Model file for the job. Use its own axes, mm. Coordinates: 2 decimals unless noted, no trailing zeros. Order: outer loops, then holes, each group sorted by start corner. A loop starts at its lowest first (then second) coordinate and runs counter-clockwise, first axis right, second up. Notation, with made-up numbers: M 62,20.25 L 112,20.25 A29 cw 112,49.25 Z; hole C 86,-26.75 d3. An arc over 180 degrees is marked long. Return JSON: item names as keys, results as strings.
```python
from build123d import *

# Parameters (mm, degrees)
SKETCH2_W           = 17
SKETCH2_H           = 5
BOSS_EXTRUDE1_DEPTH = 5
SKETCH3_R           = 1.5
SKETCH3_R_2         = 1.45
SKETCH3_R_3         = 1.55
SKETCH3_R_4         = 1.525
SKETCH3_R_5         = 1.475
CUT_EXTRUDE1_DEPTH  = 6
SKETCH4_W           = 5
SKETCH4_H           = 5
BOSS_EXTRUDE2_DEPTH = 1.5
SKETCH5_W           = 5
SKETCH5_H           = 5
BOSS_EXTRUDE3_DEPTH = 1.5
FILLET1_R           = 0.5


with BuildPart() as part:
    # Sketch2 → Boss-Extrude1 (new body)
    with BuildSketch(Plane(origin=(0, 0, 0), x_dir=(1, 0, 0), z_dir=(0, 1, 0))):
        with Locations((1.12006706, -0.094563726)):
            Rectangle(SKETCH2_W, SKETCH2_H)
    extrude(amount=BOSS_EXTRUDE1_DEPTH)

    # Sketch3 → Cut-Extrude1 (cut, through all)
    with BuildSketch(Plane(origin=(0, 5, 0), x_dir=(1, 0, 0), z_dir=(0, 1, 0))):
        with Locations((1.12006706, -0.094563726)):
            Circle(SKETCH3_R)
        with Locations((7.97006706, -0.094563726)):
            Circle(SKETCH3_R_2)
        with Locations((-5.72993294, -0.094563726)):
            Circle(SKETCH3_R_3)
        with Locations((-2.354549871, -0.094563726)):
            Circle(SKETCH3_R_4)
        with Locations((4.597069825, -0.094563726)):
            Circle(SKETCH3_R_5)
    extrude(amount=-CUT_EXTRUDE1_DEPTH, mode=Mode.SUBTRACT)

    # Sketch4 → Boss-Extrude2 (add)
    with BuildSketch(Plane.ZY.offset(7.37993294)):
        with Locations((0.094563726, 2.5)):
            Rectangle(SKETCH4_W, SKETCH4_H)
    extrude(amount=BOSS_EXTRUDE2_DEPTH)

    # Sketch5 → Boss-Extrude3 (add)
    with BuildSketch(Plane(origin=(9.62006706, 0, 0), x_dir=(0, 0, -1), z_dir=(1, 0, 0))):
        with Locations((-0.094563726, 2.5)):
            Rectangle(SKETCH5_W, SKETCH5_H)
    extrude(amount=BOSS_EXTRUDE3_DEPTH)

    # Fillet1
    fillet1_edges = [part.edges().sort_by_distance(p)[0] for p in [
        (1.12006706, 5, -2.405436274),
        (-8.87993294, 2.5, -2.405436274),
        (-8.87993294, 2.5, 2.594563726),
        (-8.87993294, 5, 0.094563726),
        (11.12006706, 2.5, 2.594563726),
        (11.12006706, 2.5, -2.405436274),
        (11.12006706, 5, 0.094563726),
        (1.12006706, 5, 2.594563726),
    ]]
    fillet(fillet1_edges, radius=FILLET1_R)


solid = part.part
```
Item 1: Pull direction Z, two halves, no side cores. Call faces 1 (the flat face through (1, 2, -2.405)), 2 (the cylindrical face through (-4.25, 2.54, -0.37)), 3 (the flat face through (1, 2, 2.595)), 4 (the flat face through (1, 0, -2)): +Z half, -Z half, draft (parallel to the pull), parting line (faces both ways), or undercut.
Check result:
{"face 1": "-Z half", "face 2": "undercut", "face 3": "+Z half", "face 4": "draft"}
Item 2: Saw through at C-C (y = 1). Write the cut outline in (x, z) (3 decimals), and give its area (3 significant figures).
Check result:
{"outline": "M -8.88,-1.905 A0.5 ccw -8.38,-2.405 L 10.62,-2.405 A0.5 ccw 11.12,-1.905 L 11.12,2.095 A0.5 ccw 10.62,2.595 L -8.38,2.595 A0.5 ccw -8.88,2.095 Z; hole C -5.73,0.095 d3.1; hole C -2.355,0.095 d3.05; hole C 1.12,0.095 d3; hole C 4.597,0.095 d2.95; hole C 7.97,0.095 d2.9", "area": "64.4 mm2"}
Item 3: Saw through at D-D (z = -1.1). Write the cut outline in (x, y), and give its area (3 significant figures).
Check result:
{"outline": "M -8.88,0 L -6.72,0 L -6.72,5 L -8.38,5 A0.5 ccw -8.88,4.5 Z; M -4.74,0 L -3.3,0 L -3.3,5 L -4.74,5 Z; M -1.41,0 L 0.21,0 L 0.21,5 L -1.41,5 Z; M 2.03,0 L 3.73,0 L 3.73,5 L 2.03,5 Z; M 5.46,0 L 7.15,0 L 7.15,5 L 5.46,5 Z; M 8.79,0 L 11.12,0 L 11.12,4.5 A0.5 ccw 10.62,5 L 8.79,5 Z", "area": "54.6 mm2"}
Item 4: Saw through at B-B (x = -2). Write the cut outline in (y, z), and give its area (3 significant figures).
Check result:
{"outline": "M 0,-2.41 L 4.5,-2.41 A0.5 ccw 5,-1.91 L 5,-1.39 L 0,-1.39 Z; M 0,1.58 L 5,1.58 L 5,2.09 A0.5 ccw 4.5,2.59 L 0,2.59 Z", "area": "10.1 mm2"}
Item 5: Saw through at A-A (z = 0.3). Write the cut outline in (x, y).
Check result:
{"outline": "M -8.88,0 L -7.27,0 L -7.27,5 L -8.38,5 A0.5 ccw -8.88,4.5 Z; M -4.19,0 L -3.87,0 L -3.87,5 L -4.19,5 Z; M -0.84,0 L -0.37,0 L -0.37,5 L -0.84,5 Z; M 2.61,0 L 3.14,0 L 3.14,5 L 2.61,5 Z; M 6.06,0 L 6.53,0 L 6.53,5 L 6.06,5 Z; M 9.41,0 L 11.12,0 L 11.12,4.5 A0.5 ccw 10.62,5 L 9.41,5 Z"}
Item 6: Wall check: line 1 (Z direction, x = 1, y = 4.2); line 2 (X direction, y = 3.95, z = -1.2); line 3 (X direction, y = 4.55, z = -1.15). Give the ranges that are in metal, low to high.
Check result:
{"line 1": "z = -2.41 to -1.4, 1.59 to 2.59", "line 2": "x = -8.88 to -6.58, -4.88 to -3.16, -1.55 to 0.36, 1.88 to 3.89, 5.3 to 7.32, 8.62 to 11.12", "line 3": "x = -8.88 to -6.65, -4.81 to -3.24, -1.47 to 0.28, 1.96 to 3.81, 5.39 to 7.23, 8.71 to 11.12"}
